Here's how the part is built. I have some questions about the finished solid (model axes, mm). A direction names the side the tool comes from. Round coordinates to 2 decimals unless told otherwise and drop trailing zeros. Order: outer loops, then holes, each group sorted by start corner. A loop starts at its lowest first (then second) coordinate and runs counter-clockwise, first axis right, second up. Notation, with made-up numbers: (55, -14.75) -> (99, -14.75) arc R8 cw to (99, -2.75) -> close; hole circle Ø10 at (-39.75, 66). An arc over 180 degrees is marked (long way). Use a Markdown table: item, result. Add a question column.
(1) If I drill on probe 1 along Y at (x, z) = (0, -18.35); probe 2 along Y at (x, z) = (-18, 17); probe 3 along X at (y, z) = (-10.5, -16), over which ranges is the centre line in solid material (lowest first)?
(2) On a 3-axis mill with a long thin cutter (end or side, diameter ignored), from which of +Z, -Z, +X, -X, +Y, -Y can I reach the whole of each face in a straight line? I mean faces 4 (the face through (-7.732, -34.818, 17.535)), 5 (the face through (2.5, -26.3, 20)), 6 (the face through (-42.452, 1.868, -17.535)). Say none if no direction works.
(3) I want a section at A-A, the plane x = 0. Please give me the cut outline in (y, z), then the cut area to 3 significant figures.
(4) Thinking about a two-plate mould opening in Y: for faces 1 (the face through (-10, 35, -15)), 2 (the face through (2.5, -26.3, -20)), 3 (the face through (-36.107, -27.686, 0.28)), which applies, pulls with the +Y half, pulls with the -Y half, needs draft (parallel to the pull), parting line crosses it, or undercut?
(5) I want a section at C-C, the plane z = 3.5. Please give me the cut outline in (x, y).
(6) I'm going to push flat-ended pins straight in: P1, Ø2, axis at x = -14.5, z = -14.5, coming from the +Y side; P2, Ø1, axis at x = -31.5, z = 7.5, coming from the -Y side; P3, Ø6, axis at x = -21.5, z = 6.5, coming from the -Y side. Where does each tip first touch, or does it pass through?
(7) I want a section at D-D, the plane y = -34.5. Please give me the cut outline in (x, z).
from build123d import *

# Parameters (mm, degrees)
SKETCH1_R           = 45.5
SKETCH1_R_2         = 26
BOSS_EXTRUDE1_DEPTH = 20
SKETCH2_R           = 42.493578565
SKETCH2_R_2         = 35.665645311
CUT_EXTRUDE2_DEPTH  = 5


with BuildPart() as part:
    # Sketch1 → Boss-Extrude1 (new body)
    with BuildSketch(Plane.XY):
        Circle(SKETCH1_R)
        Circle(SKETCH1_R_2, mode=Mode.SUBTRACT)
    boss_extrude1 = extrude(amount=BOSS_EXTRUDE1_DEPTH)

    # Sketch2 → Cut-Extrude2 (cut)
    with BuildSketch(Plane.XY.offset(20)):
        Circle(SKETCH2_R)
        Circle(SKETCH2_R_2, mode=Mode.SUBTRACT)
    cut_extrude2 = extrude(amount=-CUT_EXTRUDE2_DEPTH, mode=Mode.SUBTRACT)


with BuildPart() as mirror1_1:
    # Mirror1: Boss-Extrude1 across Front Plane
    add(boss_extrude1.mirror(Plane.XY))

    # Mirror1 2: Cut-Extrude2 across Front Plane
    add(cut_extrude2.mirror(Plane.XY), mode=Mode.SUBTRACT)


with BuildPart() as part_1:
    add(part.part)

    # Mirror1 united with what the copies touc: union Mirror1_1
    add(mirror1_1.part)


solid = part_1.part
Taken from the geometry:
| question | item | result |
|---|---|---|
| 1 | probe 1 | y = -45.5 to -42.49, -35.67 to -26, 26 to 35.67, 42.49 to 45.5 |
| 1 | probe 2 | y = -41.79 to -38.49, -30.79 to -18.76, 18.76 to 30.79, 38.49 to 41.79 |
| 1 | probe 3 | x = -44.27 to -41.18, -34.09 to -23.79, 23.79 to 34.09, 41.18 to 44.27 |
| 2 | face 4 | +Z |
| 2 | face 5 | +Z, +X, -X, +Y, -Y |
| 2 | face 6 | -Z |
| 3 | outline | (-45.5, -20) -> (-42.49, -20) -> (-42.49, -15) -> (-35.67, -15) -> (-35.67, -20) -> (-26, -20) -> (-26, 20) -> (-35.67, 20) -> (-35.67, 15) -> (-42.49, 15) -> (-42.49, 20) -> (-45.5, 20) -> close; (26, -20) -> (35.67, -20) -> (35.67, -15) -> (42.49, -15) -> (42.49, -20) -> (45.5, -20) -> (45.5, 20) -> (42.49, 20) -> (42.49, 15) -> (35.67, 15) -> (35.67, 20) -> (26, 20) -> close |
| 3 | area | 1,420 mm2 |
| 4 | face 1 | undercut |
| 4 | face 2 | needs draft |
| 4 | face 3 | parting line crosses it |
| 5 | outline | circle Ø91 at (0, 0); hole circle Ø52 at (0, 0) |
| 6 | P1 | stops at y = 43.45 |
| 6 | P2 | stops at y = -33.31 |
| 6 | P3 | stops at y = -41.57 |
| 7 | outline | (-29.66, -20) -> (-24.81, -20) -> (-24.81, -15) -> (-9.04, -15) -> (-9.04, -20) -> (9.04, -20) -> (9.04, -15) -> (24.81, -15) -> (24.81, -20) -> (29.66, -20) -> (29.66, 20) -> (24.81, 20) -> (24.81, 15) -> (9.04, 15) -> (9.04, 20) -> (-9.04, 20) -> (-9.04, 15) -> (-24.81, 15) -> (-24.81, 20) -> (-29.66, 20) -> close |
